from build123d import *

# Parameters (mm, degrees)
SM_BASE_FLANGE_1_DEPTH   = 45
SKETCH_7_R               = 13
CUT_EXTRUDE_1_DEPTH      = 63.841069373
CHAMFER_1_SIZE           = 10
SKETCH_9_R               = 1
CUT_EXTRUDE_3_DEPTH      = 82.541400528
M5X0_8_1_D               = 4.2
CUT_EXTRUDE_4_REACH      = 64.841
SKETCH_11_R              = 1.7
PATTERN_CIRCULAR_1_COUNT = 4


# Sheet-metal steps are written as plain solids
with BuildPart() as part:
    # Sketch 2 → 基材-凸緣1 (new, symmetric)
    with BuildSketch(Plane(origin=(0, 0, 0), x_dir=(0, 0, -1), z_dir=(1, 0, 0))):
        with BuildLine():
            Line((32, -30), (5.5, -30))
            ThreePointArc((5.5, -30), (1.610912703, -28.389087297), (0, -24.5))
            Line((0, -24.5), (0, 24.5))
            ThreePointArc((0, 24.5), (1.610912703, 28.389087297), (5.5, 30))
            Line((5.5, 30), (32, 30))
            Line((32, 30), (32, 26))
            Line((32, 26), (5.5, 26))
            ThreePointArc((5.5, 26), (4.439339828, 25.560660172), (4, 24.5))
            Line((4, 24.5), (4, -24.5))
            ThreePointArc((4, -24.5), (4.439339828, -25.560660172), (5.5, -26))
            Line((5.5, -26), (32, -26))
            Line((32, -26), (32, -30))
        make_face()
    extrude(amount=SM_BASE_FLANGE_1_DEPTH, both=True)

    # 草圖7 → 除料-伸長1 (cut, through all)
    with BuildSketch(Plane.XY):
        with Locations((0, -3)):
            Circle(SKETCH_7_R)
    extrude(amount=-CUT_EXTRUDE_1_DEPTH, mode=Mode.SUBTRACT)

    # 導角1
    chamfer_1_edges = [part.edges().sort_by_distance(p)[0] for p in [
        (-45, 28, -32),
        (-45, -28, -32),
        (45, 28, -32),
        (45, -28, -32),
    ]]
    chamfer(chamfer_1_edges, length=CHAMFER_1_SIZE)

    # 草圖9 → 除料-伸長3 (cut, through all)
    with BuildSketch(Plane(origin=(0, 30, 0), x_dir=(1, 0, 0), z_dir=(0, 1, 0))):
        with Locations(Location((-27.5, 24, 0), (0, 0, 270))):
            Circle(SKETCH_9_R)
        with Locations(Location((27.5, 24, 0), (0, 0, 270))):
            Circle(SKETCH_9_R)
        with Locations(Location((-27.5, 12, 0), (0, 0, 270))):
            Circle(SKETCH_9_R)
        with Locations(Location((27.5, 12, 0), (0, 0, 270))):
            Circle(SKETCH_9_R)
    extrude(amount=-CUT_EXTRUDE_3_DEPTH, mode=Mode.SUBTRACT)

    # M5x0.8 螺紋孔1 (through all)
    with Locations(Plane(origin=(-27.5, 30, -24), x_dir=(0, 0, 1), z_dir=(0, 1, 0))):
        with Locations((0, 0), (12, 0), (12, 55), (0, 55)):
            Hole(M5X0_8_1_D / 2)

    # 草圖11 → 除料-伸長4 (cut, up to next)
    with BuildSketch(Plane.XY, mode=Mode.PRIVATE) as cut_extrude_4_sk1:
        with Locations((-16.970562748, 13.970562748)):
            Circle(SKETCH_11_R)
    cut_extrude_4_tool1 = extrude(cut_extrude_4_sk1.sketch, amount=-CUT_EXTRUDE_4_REACH, mode=Mode.PRIVATE) & part.part
    cut_extrude_4 = cut_extrude_4_tool1.solids().sort_by_distance((-16.970563, 13.970563, 0))[0]
    add(cut_extrude_4, mode=Mode.SUBTRACT)

    # 環狀複製排列1: 除料-伸長4 ×4 about axis
    pattern_circular_1_axis = Axis((0, -3, 0), (0, 0, 1))
    for i in range(1, PATTERN_CIRCULAR_1_COUNT):
        add(cut_extrude_4.rotate(pattern_circular_1_axis, i * 360 / PATTERN_CIRCULAR_1_COUNT), mode=Mode.SUBTRACT)


solid = part.part
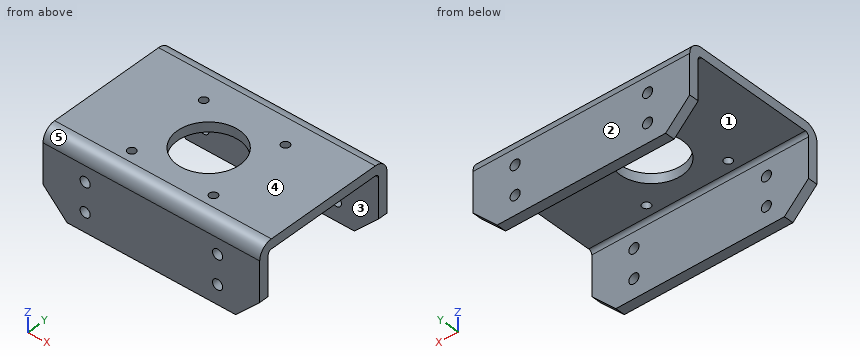
Source: CAD feature listing. Evaluate the final solid. Frame: model axes, mm. Face numbers are marked on the shaded views. A direction names the side the tool comes from. Round coordinates to 2 decimals unless told otherwise and drop trailing zeros. Loops run counter-clockwise (first coordinate to the right, second up) from the corner with the lowest first, then second, coordinate; pieces in that order, holes last. Notation, with made-up numbers: (59, 51) - (118, 51) arc R20 ccw to (118, 66) - close; hole circle Ø2 at (75, 89.5). An arc over 180 degrees is marked (long way). Write item = value, one per line. Start each with the question number.
(1) Section query A-A, the plane y = -3. Output: boundary loops of the cut face in (x, z), plus the area to 3 significant figures.
(2) Pin query (flat end, axial travel): pin 1 (4 mm diameter, centred on x = 27.5, z = -12, fed in from -Y); pin 2 (12 mm diameter, centred on x = 22, y = 9.5, fed in from -Z). Return the tip coordinate at first contact, or that it passes through.
(3) Section query C-C, the plane z = -6.5. Output: boundary loops of the cut face in (x, y).
(4) Pull-direction query (Y, two-part tool) for the marked faces 3, 4 and 5; classes: +Y half, -Y half, draft (parallel to the pull), parting line (faces both ways), or undercut.
(5) Ray query, line 1 along X through (y, z) = (-27.1, -12); line 2 along Y through (x, z) = (-35.5, -26.5); line 3 along X through (y, z) = (28, -24). Return the intervals inside material, ascending. Write a range as from..to.
(6) Set-up query: the marked faces 1 and 2. Return all of +Z, -Z, +X, -X, +Y, -Y with unobstructed straight access to the full face (end or side cutting, diameter ignored); none if empty.
(7) Section query D-D, the plane x = -27.5. Output: boundary loops of the cut face in (y, z).
(8) Section query B-B, the plane z = -24. Output: boundary loops of the cut face in (x, y), plus the area to 3 significant figures.
Conclusion:
q1.outline = (-45, -4) - (-13, -4) - (-13, 0) - (-45, 0) - close; (13, -4) - (45, -4) - (45, 0) - (13, 0) - close
q1.area = 256 mm2
q2.pin_1 = through
q2.pin_2 = -4
q3.outline = (-45, -30) - (45, -30) - (45, -26) - (-45, -26) - close; (-45, 26) - (45, 26) - (45, 30) - (-45, 30) - close
q4.face_3 = undercut
q4.face_4 = draft
q4.face_5 = -Y half
q5.line_1 = -45..-29.6, -25.4..25.4, 29.6..45
q5.line_2 = -30..-26, 26..30
q5.line_3 = -43..-29.6, -25.4..25.4, 29.6..43
q6.face_1 = -Z, +X, -X
q6.face_2 = +Z, -Z, +X, -X, +Y
q7.outline = (-30, -32) - (-26, -32) - (-26, -26.1) - (-30, -26.1) - close; (-30, -21.9) - (-26, -21.9) - (-26, -14.1) - (-30, -14.1) - close; (-30, -9.9) - (-26, -9.9) - (-26, -5.5) arc R1.5 cw to (-24.5, -4) - (24.5, -4) arc R1.5 cw to (26, -5.5) - (26, -9.9) - (30, -9.9) - (30, -5.5) arc R5.5 ccw to (24.5, 0) - (-24.5, 0) arc R5.5 ccw to (-30, -5.5) - close; (26, -32) - (30, -32) - (30, -26.1) - (26, -26.1) - close; (26, -21.9) - (30, -21.9) - (30, -14.1) - (26, -14.1) - close
q8.outline = (-43, -30) - (-29.6, -30) - (-29.6, -26) - (-43, -26) - close; (-43, 26) - (-29.6, 26) - (-29.6, 30) - (-43, 30) - close; (-25.4, -30) - (25.4, -30) - (25.4, -26) - (-25.4, -26) - close; (-25.4, 26) - (25.4, 26) - (25.4, 30) - (-25.4, 30) - close; (29.6, -30) - (43, -30) - (43, -26) - (29.6, -26) - close; (29.6, 26) - (43, 26) - (43, 30) - (29.6, 30) - close
q8.area = 621 mm2
